```python
from build123d import *

# Parameters (mm, degrees)
SKETCH1_R           = 5.1435
SKETCH1_R_2         = 1.524
BOSS_EXTRUDE1_DEPTH = 3.175
SKETCH2_R           = 0.762
CUT_EXTRUDE1_DEPTH  = 3.175
CIRPATTERN1_COUNT   = 6


with BuildPart() as part:
    # Sketch1 → Boss-Extrude1 (new body)
    with BuildSketch(Plane.XY):
        Circle(SKETCH1_R)
        Circle(SKETCH1_R_2, mode=Mode.SUBTRACT)
    extrude(amount=BOSS_EXTRUDE1_DEPTH)

    # Sketch2 → Cut-Extrude1 (cut)
    with BuildSketch(Plane.XY.offset(3.175)):
        with Locations((0, 3.33375)):
            Circle(SKETCH2_R)
    cut_extrude1 = extrude(amount=-CUT_EXTRUDE1_DEPTH, mode=Mode.SUBTRACT)

    # CirPattern1: Cut-Extrude1 ×6 about axis
    cirpattern1_axis = Axis((0, 0, 0), (0, 0, 1))
    for i in range(1, CIRPATTERN1_COUNT):
        add(cut_extrude1.rotate(cirpattern1_axis, i * 360 / CIRPATTERN1_COUNT), mode=Mode.SUBTRACT)


solid = part.part
```
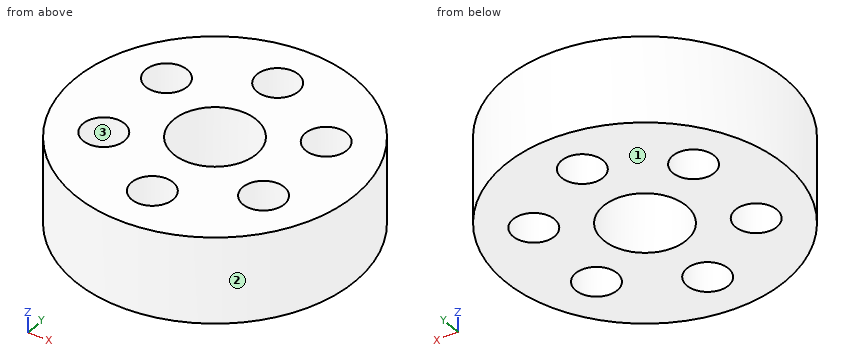
Verification items for the finished model (mm, model axes). Face numbers are marked on the shaded views. Coordinates: 2 decimals unless noted, no trailing zeros. Loops run counter-clockwise (first coordinate to the right, second up) from the corner with the lowest first, then second, coordinate; pieces in that order, holes last. Notation, with made-up numbers: (9, 33.5) -> (44, 33.5) arc R24 cw to (44, 65.5) -> close; hole circle Ø1 at (60.25, 20.5). An arc over 180 degrees is marked (long way). Answer in a Markdown table with one row per item.
1) Draft check along Y on the marked faces 1, 2 and 3. Enter one of: released by +Y, released by -Y, zero draft, split by the parting line, or undercut.
The answers:
| item | result |
|---|---|
| face 1 | zero draft |
| face 2 | split by the parting line |
| face 3 | undercut |
2) Section check B-B (y = 0). Record the cut outline in (x, z) (1 decimal).
The answers:
| item | result |
|---|---|
| outline | (-5.1, 0) -> (-1.5, 0) -> (-1.5, 3.2) -> (-5.1, 3.2) -> close; (1.5, 0) -> (5.1, 0) -> (5.1, 3.2) -> (1.5, 3.2) -> close |
3) Section check A-A (x = 0). Record the cut outline in (y, z) (1 decimal).
The answers:
| item | result |
|---|---|
| outline | (-5.1, 0) -> (-4.1, 0) -> (-4.1, 3.2) -> (-5.1, 3.2) -> close; (-2.6, 0) -> (-1.5, 0) -> (-1.5, 3.2) -> (-2.6, 3.2) -> close; (1.5, 0) -> (2.6, 0) -> (2.6, 3.2) -> (1.5, 3.2) -> close; (4.1, 0) -> (5.1, 0) -> (5.1, 3.2) -> (4.1, 3.2) -> close |
4) Section check D-D (z = 0.95). Record the cut outline in (x, y).
The answers:
| item | result |
|---|---|
| outline | circle Ø10.29 at (0, 0); hole circle Ø1.52 at (-2.89, -1.67); hole circle Ø1.52 at (-2.89, 1.67); hole circle Ø3.05 at (0, 0); hole circle Ø1.52 at (0, -3.33); hole circle Ø1.52 at (0, 3.33); hole circle Ø1.52 at (2.89, -1.67); hole circle Ø1.52 at (2.89, 1.67) |
5) Section check C-C (x = 2.75). Record the cut outline in (y, z) (3 decimals), and give its area (3 significant figures).
The answers:
| item | result |
|---|---|
| outline | (-4.347, 0) -> (-2.416, 0) -> (-2.416, 3.175) -> (-4.347, 3.175) -> close; (-0.917, 0) -> (0.917, 0) -> (0.917, 3.175) -> (-0.917, 3.175) -> close; (2.416, 0) -> (4.347, 0) -> (4.347, 3.175) -> (2.416, 3.175) -> close |
| area | 18.1 mm2 |
6) Scan lines: line 1 along Y through (x, z) = (0, 1.4); line 2 along Y through (x, z) = (3, 2.95); line 3 along Y through (x, z) = (2.5, 0.9). Record each from-to range of solid material in increasing order. Write a range as from..to.
The answers:
| item | result |
|---|---|
| line 1 | y = -5.14..-4.1, -2.57..-1.52, 1.52..2.57, 4.1..5.14 |
| line 2 | y = -4.18..-2.42, -0.91..0.91, 2.42..4.18 |
| line 3 | y = -4.5..-2.32, -1.01..1.01, 2.32..4.5 |
